```python
from build123d import *

# Parameters (mm, degrees)
BOSS_EXTRUDE1_DEPTH = 0.515
SKETCH2_R           = 5.5
BOSS_EXTRUDE2_DEPTH = 0.01
SKETCH3_R           = 3.75
BOSS_EXTRUDE5_DEPTH = 0.525
BOSS_EXTRUDE6_DEPTH = 0.01
SKETCH6_R           = 0.5
CUT_EXTRUDE1_DEPTH  = 96.72347361
LPATTERN1_COUNT     = 15
LPATTERN1_PITCH     = 2.55
SKETCH7_R           = 2.275
SKETCH7_R_2         = 1.25
CUT_EXTRUDE2_DEPTH  = 96.72347361


with BuildPart() as part:
    # Sketch1 → Boss-Extrude1 (new, symmetric)
    with BuildSketch(Plane.XY):
        with BuildLine():
            Line((0, 0), (55.75, 0))
            Line((55.75, 0), (58.15, 1.25))
            Line((58.15, 1.25), (81.25, 1.25))
            Line((81.25, 1.25), (81.25, -37.85))
            Line((81.25, -37.85), (65.45, -37.85))
            ThreePointArc((65.45, -37.85), (56.43438854, -41.58438854), (52.7, -50.6))
            Line((52.7, -50.6), (21.8, -50.6))
            Line((21.8, -50.6), (21.8, -41.4))
            Line((21.8, -41.4), (19.042567568, -38.75))
            Line((19.042567568, -38.75), (8.792567568, -38.75))
            Line((8.792567568, -38.75), (0, -30.3))
            Line((0, -30.3), (0, 0))
        make_face()
    extrude(amount=BOSS_EXTRUDE1_DEPTH, both=True)

    # Sketch2 → Boss-Extrude2 (add)
    with BuildSketch(Plane.XY.offset(0.515)):
        with Locations(Location((66.25, -4.5, 0), (0, 0, 180))):
            Circle(SKETCH2_R)
        with Locations(Location((73.15, -18.935719587, 0), (0, 0, 180))):
            Circle(SKETCH2_R)
        with Locations(Location((58.696235763, -25.844344587, 0), (0, 0, 180))):
            Circle(SKETCH2_R)
        with Locations(Location((51.796235763, -11.408625, 0), (0, 0, 180))):
            Circle(SKETCH2_R)
    extrude(amount=BOSS_EXTRUDE2_DEPTH)

    # Sketch3 → Boss-Extrude5 (add, through all)
    with BuildSketch(Plane.XY):
        with Locations((15, -14.375)):
            Circle(SKETCH3_R)
        with Locations((15, -32.625)):
            Circle(SKETCH3_R)
        with Locations((24.125, -23.5)):
            Circle(SKETCH3_R)
        with Locations((5.875, -23.5)):
            Circle(SKETCH3_R)
    extrude(amount=BOSS_EXTRUDE5_DEPTH)

    # Sketch5 → Boss-Extrude6 (add)
    with BuildSketch(Plane.XY.offset(0.515)):
        Polygon((32.918861679, -40.773499762), (23.3, -45.573499762), (25.309302326, -49.6), (34.928164005, -44.8), align=None)
        Polygon((38.3, -45.573499762), (40.309302326, -49.6), (49.928164005, -44.8), (47.918861679, -40.773499762), align=None)
    extrude(amount=BOSS_EXTRUDE6_DEPTH)

    # Sketch6 → Cut-Extrude1 (cut, through all)
    with BuildSketch(Plane.XY.offset(0.515)):
        with Locations((57.25, -1)):
            Circle(SKETCH6_R)
    cut_extrude1 = extrude(amount=-CUT_EXTRUDE1_DEPTH, mode=Mode.SUBTRACT)

    # LPattern1: Cut-Extrude1 ×15
    with Locations(*[(-i * LPATTERN1_PITCH, 0, 0) for i in range(1, LPATTERN1_COUNT)]):
        add(cut_extrude1, mode=Mode.SUBTRACT)

    # Sketch7 → Cut-Extrude2 (cut, through all)
    with BuildSketch(Plane.XY.offset(0.515)):
        with Locations((67.5, -34.1)):
            Circle(SKETCH7_R)
        with Locations((78.5, -31)):
            Circle(SKETCH7_R_2)
    extrude(amount=-CUT_EXTRUDE2_DEPTH, mode=Mode.SUBTRACT)


solid = part.part
```
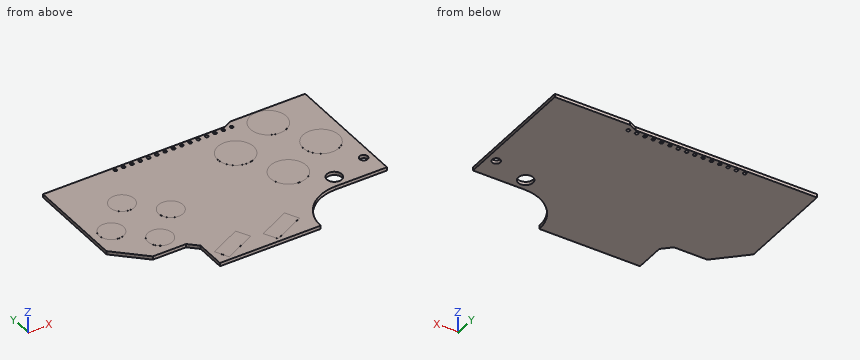
Can you work these out from the model? Positions are in its coordinate system, mm. Round coordinates to 2 decimals unless told otherwise and drop trailing zeros. Order: outer loops, then holes, each group sorted by start corner. A loop starts at its lowest first (then second) coordinate and runs counter-clockwise, first axis right, second up. Notation, with made-up numbers: (62.5, 7) -> (94.5, 7) arc R15 cw to (94.5, 27) -> close; hole circle Ø5 at (33.5, 0.25). An arc over 180 degrees is marked (long way). Return JSON: item names as keys, results as strings. Group by question number.
1. I need wall thicknesses on line 1 (Y direction, x = 36.85, z = 0.05); line 2 (Y direction, x = 78.5, z = 0.3); line 3 (Y direction, x = 18, z = 0.15). Which ranges of each line are inside material? Lowest first, please. Write a range as [from, to].
2. Will these pins go through, and if not, where does the flat tip stop? pin 1 (7.5 mm diameter, centred on x = 67.5, y = -34.1, fed in from -Z) (3 decimals); pin 2 (2 mm diameter, centred on x = 78.5, y = -31, fed in from -Z); pin 3 (1.5 mm diameter, centred on x = 62.5, y = -20.5, fed in from +Z) (3 decimals).
3. If we section it at D-D, the plane y = -40: Write out the boundary of the cut face in (x, z) (3 decimals), then the cut area to 3 significant figures.
4. If we section it at B-B, the plane y = -34.1: Write out the boundary of the cut face in (x, z) (3 decimals).
5. If we section it at A-A, the plane z = 0.35: Count the separate pieces of the cut face and the enclosed holes in it, then the cut area to 3 significant figures.
6. If we section it at C-C, the plane x = 73.15: Write out the boundary of the cut face in (y, z) (3 decimals), then the cut area to 3 significant figures.
Output values:
{
 "1": {"line 1": "[-50.6, -1.5], [-0.5, 0]", "line 2": "[-37.85, -32.25], [-29.75, 1.25]", "line 3": "[-38.75, 0]"},
 "2": {"pin 1": "z = -0.515", "pin 2": "through", "pin 3": "z = 0.515"},
 "3": {"outline": "(20.343, -0.515) -> (58.365, -0.515) -> (58.365, 0.515) -> (20.343, 0.515) -> close", "area": "39.2 mm²"},
 "4": {"outline": "(3.954, -0.515) -> (65.225, -0.515) -> (65.225, 0.515) -> (18.448, 0.515) -> (18.448, 0.525) -> (11.552, 0.525) -> (11.552, 0.515) -> (3.954, 0.515) -> close; (69.775, -0.515) -> (81.25, -0.515) -> (81.25, 0.515) -> (69.775, 0.515) -> close"},
 "5": {"separate pieces": "1", "enclosed holes": "17", "area": "3,490 mm²"},
 "6": {"outline": "(-37.85, -0.515) -> (1.25, -0.515) -> (1.25, 0.515) -> (-13.436, 0.515) -> (-13.436, 0.525) -> (-24.436, 0.525) -> (-24.436, 0.515) -> (-37.85, 0.515) -> close", "area": "40.4 mm²"}
}
